Geometry check sheet. Reference: drawing and pictorial views, mm from the part's lowest x, y, z. A direction names the side the tool comes from. Give positions to 0.01 mm unless a question says otherwise; leave off trailing zeros. Order: outer loops, then holes, each group sorted by start corner. A loop starts at its lowest first (then second) coordinate and runs counter-clockwise, first axis right, second up.
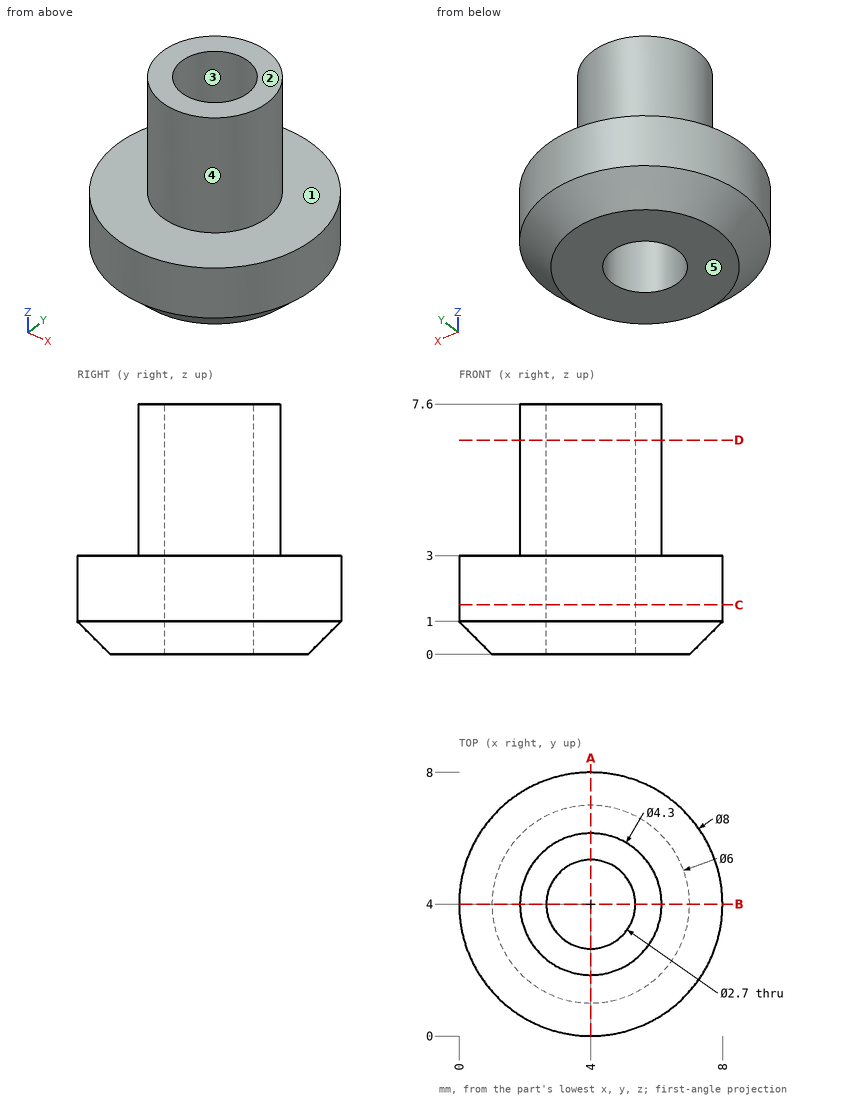
(1) Set-up check for the marked faces 1 and 2: record each of +Z, -Z, +X, -X, +Y, -Y from which the full face is reachable in a straight line by a thin tool's end or side.
Response values:
face 1: +Z
face 2: +Z, +X, -X, +Y, -Y
(2) Cross-section at D-D on z = 6.5. Enter the section's corners in (x, y).
Response values:
outline: circle Ø4.3 at (4, 4); hole circle Ø2.7 at (4, 4)
(3) Cross-section at C-C on z = 1.5. Enter the section's corners in (x, y), then the cut area to 3 significant figures.
Response values:
outline: circle Ø8 at (4, 4); hole circle Ø2.7 at (4, 4)
area: 44.5 mm2
(4) Release check for a two-part mould opening along Y. For the marked faces 3, 4 and 5 record: released by +Y, released by -Y, zero draft, split by the parting line, or undercut.
Response values:
face 3: undercut
face 4: split by the parting line
face 5: zero draft
(5) Material ranges on L1, parallel to Y at x = 4, z = 6.25; L2, parallel to Z at x = 3, y = 2; L3, parallel to X at y = 3.25, z = 2, recorded low to high.
Response values:
L1: y = 1.85 to 2.65, 5.35 to 6.15
L2: z = 0 to 3
L3: x = 0.07 to 2.88, 5.12 to 7.93
(6) Gauge pin test, flat ends, axial feed: pin 1 Ø2 at (y, z) = (2.5, 5.5) entering from +X; pin 2 Ø1 at (y, z) = (3, 4.5) entering from -X. Record the tip position at first contact, or that the pin passes through.
Response values:
pin 1: stops at x = 6.09
pin 2: stops at x = 1.91
(7) Cross-section at A-A on x = 4. Enter the section's corners in (y, z), then the cut area to 3 significant figures.
Response values:
outline: (0, 1) - (1, 0) - (2.65, 0) - (2.65, 7.6) - (1.85, 7.6) - (1.85, 3) - (0, 3) - close; (5.35, 0) - (7, 0) - (8, 1) - (8, 3) - (6.15, 3) - (6.15, 7.6) - (5.35, 7.6) - close
area: 22.3 mm2
